from build123d import *

# Parameters (mm, degrees)
F1_DEPTH = 4.318


with BuildPart() as f1:
    # F0 (on Top) → F1 (new body)
    with BuildSketch(Plane.XY):
        with BuildLine():
            add(Edge.make_bspline(
                [(0, 38.7419006444), (0, 40.780224347), (4.0504073247, 43.2264357913), (13.3197663427, 47.2353910075), (23.679706238, 49.0470707989), (29.4917598367, 49.0470707989)],
                knots=[0, 0, 0, 0, 0.243800261, 0.5764746481, 1, 1, 1, 1], degree=3))
            Line((0, 38.7419006444), (0, 0))
            Line((0, 0), (749.3, 0))
            Line((749.3, 0), (749.3, 9.525))
            Line((749.3, 9.525), (477.4143925697, 35.56))
            Line((477.4143925697, 35.56), (172.9129329324, 49.0470707989))
            Line((172.9129329324, 49.0470707989), (29.4917598367, 49.0470707989))
        make_face()
    extrude(amount=F1_DEPTH)


solid = f1.part
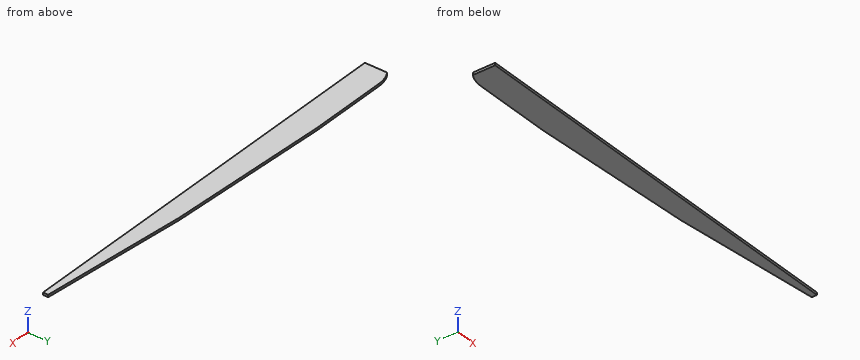
Geometry: final body of the model. Coordinates: model frame, mm. Coordinates: 2 decimals unless noted, no trailing zeros. Order: outer loops, then holes, each group sorted by start corner. A loop starts at its lowest first (then second) coordinate and runs counter-clockwise, first axis right, second up.
1) Section B-B (y = 22.5). Return loops of the section in (x, z).
Result sheet:
outline: (0, 0) - (613.8, 0) - (613.8, 4.32) - (0, 4.32) - close
2) Ray query, probe 1 along Y at (x, z) = (251.5, 3.3); probe 2 along Y at (x, z) = (254, 0.5). Return the intervals inside material, ascending.
Result sheet:
probe 1: y = 0 to 45.57
probe 2: y = 0 to 45.46
3) Section A-A (x = 200). Return loops of the section in (y, z).
Result sheet:
outline: (0, 0) - (47.85, 0) - (47.85, 4.32) - (0, 4.32) - close
4) First-contact query: P1, Ø2, axis at x = 291.5, z = 0.5, coming from the +Y side. Flat tip, straight axial feed; report the tip coordinate or a pass-through.
Result sheet:
P1: stops at y = 43.84
